CAD build for the part. Positions are in the model's coordinates, mm. Face numbers are marked on the shaded views. A direction names the side the tool comes from. Give positions to 0.01 mm unless a question says otherwise; leave off trailing zeros. Write each loop counter-clockwise with the first axis right and the second up, starting at its lowest first coordinate (ties: lowest second). Pieces come first, ordered by that corner, then holes. Notation, with made-up numbers: (35.25, 35) - (57.25, 35) arc R29 cw to (57.25, 72) - close; hole circle Ø10 at (42, 65.5). An arc over 180 degrees is marked (long way). Put each result on its own line as item: value. Start each with the question number.
1. Drop flat-ended pins along their axis: pin 1 (6 mm diameter, centred on y = 28.5, z = -41, fed in from +X); pin 2 (4 mm diameter, centred on x = 31.5, y = 64.5, fed in from +Z); pin 3 (8 mm diameter, centred on x = 10, y = 44, fed in from -Z); pin 4 (24.5 mm diameter, centred on y = 0, z = 0, fed in from -X). Give the stop position or say it passes through.
2. Cut at A-A on x = 12.5. List the corners of the cut face in (y, z).
3. Cut at C-C on x = 67. List the corners of the cut face in (y, z), and give its area (3 significant figures).
4. Tool access for the marked faces 4, 5 and 6: list every direction of +Z, -Z, +X, -X, +Y, -Y with a clear straight run to the whole face (end or side of a thin tool).
5. Wall check: line 1 (X direction, y = 15, z = 0); line 2 (Z direction, x = 5, y = 13.5) (3 decimals); line 3 (Z direction, x = 18.5, y = 30). Give the ranges that are in metal, low to high.
6. Mould opens along Z. For the marked faces 1, 2 and 3 say: +Z half, -Z half, draft (parallel to the pull), parting line (faces both ways), or undercut.
7. Cut at B-B on z = 0. Give the number of separate pieces and of enclosed holes in the cut face, and give its area (3 significant figures).
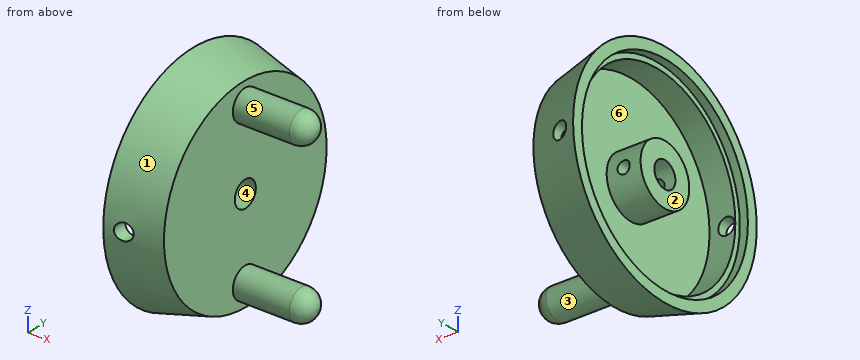
Autodesk Inventor part; units mm, degrees
ref_plane "Work Plane1" through (12.5, 22, 0) normal (0, 1, 0) x (-1, 0, 0)
ref_plane "Work Plane2" through (12.5, -22, 0) normal (0, 1, 0) x (-1, 0, 0)
ref_plane "YZ Plane" through (0, 0, 0) normal (1, 0, 0) x (0, 1, 0)
sketch "Sketch1" plane through (0, 0, 0) normal (0, 0, 1) x (1, 0, 0)
  line L0 (0, 0) -> (0, 22)
  line L1 (0, 22) -> (25, 22)
  line L2 (25, 22) -> (25, 71)
  line L3 (25, 71) -> (6, 71)
  line L4 (6, 71) -> (6, 75)
  line L5 (6, 75) -> (0, 75)
  line L6 (37, 0) -> (37, 73.5)
  line L7 (0, 75) -> (0, 83)
  line L8 (0, 83) -> (37, 73.5)
  line L9 (0, 0) -> (37, 0)
  dimension "d0" = 22
  dimension "d1" = 25
  dimension "d2" = 49
  dimension "d3" = 19
  dimension "d4" = 4
  dimension "d6" = 37
  dimension "d7" = 73.5
  dimension "d8" = 8
  dimension "d9" = 104.4
revolve "Revolution1" add sketch "Sketch1" angle 360 about axis through (0, 0, 0) along (1, 0, 0)
sketch "Sketch2" plane through (0, 0, 0) normal (-1, 0, 0) x (0, 0, 1)
  circle A0 centre (0, 0) radius 9.5
  dimension "d11" = 19
extrude "Extrusion1" cut sketch "Sketch2" against normal blind 37
sketch "Sketch3" plane through (37, 0, 0) normal (1, 0, 0) x (0, 0, -1)
  point P0 (0, 0)
sketch "Sketch4" plane through (25, 0, 0) normal (-1, 0, 0) x (0, 0, 1)
  point P0 (0, 0)
ref_plane "Work Plane1" through (12.5, 22, 0) normal (0, 1, 0) x (-1, 0, 0)
sketch "Sketch5" plane through (12.5, 22, 0) normal (0, 1, 0) x (-1, 0, 0)
  point P0 (12.5, 0)
  point P1 (0, 0)
  point P2 (0, 0)
  point P3 (0, 0)
sketch "Sketch6" plane through (37, 0, 0) normal (1, 0, 0) x (0, 0, -1)
  circle A0 centre (-57.5, 0) radius 11.25
  circle A1 centre (57.5, 0) radius 11.25
  point P0 (0, 0)
  dimension "d15" = 22.5
  dimension "d16" = 22.5
extrude "Extrusion2" add sketch "Sketch6" along normal blind 52.5
fillet "Fillet1" radius 11 2 edges at (89.5, 0, 68.75) (89.5, 0, -46.25)
hole "Hole1" at (12.5, 22, 0) direction (0, -1, 0) diameter 9 depth 45 tip angle 118
sketch "Sketch7" plane through (12.5, 22, 0) normal (0, 1, 0) x (-1, 0, 0)
  point P0 (12.5, 0)
  point P1 (0, 0)
  point P2 (0, 0)
hole "Hole2" at (12.5, 22, 0) direction (0, 1, 0) diameter 12 end through all
ref_plane "Work Plane2" through (12.5, -22, 0) normal (0, 1, 0) x (-1, 0, 0)
sketch "Sketch8" plane through (12.5, -22, 0) normal (0, 1, 0) x (-1, 0, 0)
  point P0 (12.5, 0)
  point P1 (0, 0)
  point P2 (0, 0)
hole "Hole3" at (12.5, -22, 0) direction (0, -1, 0) diameter 12 end through all
properties part number "volante final"
Report:
1. pin 1: stops at x = 37
1. pin 2: stops at z = 41.44
1. pin 3: stops at z = -70.07
1. pin 4: stops at x = 0
2. outline: (-79.56, -6) arc R79.79 ccw to (79.56, -6) - (70.75, -6) arc R71 cw to (-70.75, -6) - close; (-79.56, 6) - (-70.75, 6) arc R71 cw to (70.75, 6) - (79.56, 6) arc R79.79 ccw to start; (-21.53, -4.5) arc R22 ccw to (21.53, -4.5) - (8.37, -4.5) arc R9.5 cw to (-8.37, -4.5) - close; (-21.53, 4.5) - (-8.37, 4.5) arc R9.5 cw to (8.37, 4.5) - (21.53, 4.5) arc R22 ccw to start
3. outline: circle Ø22.5 at (0, -57.5); circle Ø22.5 at (0, 57.5)
3. area: 795 mm²
4. face 4: +X, -X
4. face 5: +X
4. face 6: -X
5. line 1: x = 0 to 8, 17 to 37
5. line 2: z = -80.593 to -73.775, -17.371 to 17.371, 73.775 to 80.593
5. line 3: z = -72.27 to -64.35, 64.35 to 72.27
6. face 1: parting line
6. face 2: draft
6. face 3: undercut
7. separate pieces: 6
7. enclosed holes: 0
7. area: 2,150 mm²
